```python
from build123d import *

# Parameters (mm, degrees)
EXTRUDE_3_DEPTH = 10
EXTRUDE_4_DEPTH = 20
SKETCH_6_W      = 120
SKETCH_6_H      = 120
EXTRUDE_5_DEPTH = 30


with BuildPart() as part:
    # 草圖1 → 填料-伸長3 (new body)
    with BuildSketch(Plane(origin=(0, 0, 0), x_dir=(1, 0, 0), z_dir=(0, 1, 0))):
        with BuildLine():
            Line((-60, 50), (60, 50))
            ThreePointArc((60, 50), (110, 0), (60, -50))
            Line((60, -50), (-60, -50))
            ThreePointArc((-60, -50), (-110, 0), (-60, 50))
        make_face()
        with BuildLine():
            Line((-60, -30), (60, -30))
            ThreePointArc((60, -30), (90, 0), (60, 30))
            Line((60, 30), (-60, 30))
            ThreePointArc((-60, 30), (-90, 0), (-60, -30))
        make_face(mode=Mode.SUBTRACT)
    extrude(amount=EXTRUDE_3_DEPTH)

    # 草圖4 → 填料-伸長4 (add)
    # profile 1 of 2: a face of its own
    with BuildSketch(Plane(origin=(0, 0, 0), x_dir=(1, 0, 0), z_dir=(0, 1, 0))):
        with BuildLine():
            Line((-60, 50), (60, 50))
            ThreePointArc((60, 50), (110, 0), (60, -50))
            Line((60, -50), (-60, -50))
            ThreePointArc((-60, -50), (-110, 0), (-60, 50))
        make_face()
        with BuildLine():
            ThreePointArc((60, -47), (107, 0), (60, 47))
            Line((60, 47), (-60, 47))
            ThreePointArc((-60, 47), (-107, 0), (-60, -47))
            Line((-60, -47), (60, -47))
        make_face(mode=Mode.SUBTRACT)
    # profile 2 of 2: a face of its own
    with BuildSketch(Plane(origin=(0, 0, 0), x_dir=(1, 0, 0), z_dir=(0, 1, 0))):
        with BuildLine():
            Line((-60, 33), (60, 33))
            ThreePointArc((60, 33), (93, 0), (60, -33))
            Line((60, -33), (-60, -33))
            ThreePointArc((-60, -33), (-93, 0), (-60, 33))
        make_face()
        with BuildLine():
            ThreePointArc((-60, 30), (-90, 0), (-60, -30))
            Line((-60, -30), (60, -30))
            ThreePointArc((60, -30), (90, 0), (60, 30))
            Line((60, 30), (-60, 30))
        make_face(mode=Mode.SUBTRACT)
    extrude(amount=EXTRUDE_4_DEPTH)

    # 草圖6 → 填料-伸長5 (add)
    with BuildSketch(Plane(origin=(0, 0, 0), x_dir=(1, 0, 0), z_dir=(0, 1, 0))):
        Rectangle(SKETCH_6_W, SKETCH_6_H)
    extrude(amount=-EXTRUDE_5_DEPTH)


solid = part.part
```
Verification items for the finished model (mm, model axes). A direction names the side the tool comes from. Coordinates: 2 decimals unless noted, no trailing zeros. Order: outer loops, then holes, each group sorted by start corner. A loop starts at its lowest first (then second) coordinate and runs counter-clockwise, first axis right, second up. Notation, with made-up numbers: (51.5, 24) -> (62.5, 24) arc R34 cw to (62.5, 61) -> close; hole circle Ø7 at (0.5, 27). An arc over 180 degrees is marked (long way). Put each result on its own line as item: value. Start each with the question number.
1) Cross-section at D-D (x = -49.5). Enter the section's corners in (y, z), plus the area to 3 significant figures.
2) Release check for a two-part mould opening along X. For faces 1 (the flat face through (-60, -15, 1)), 2 (the cylindrical face through (106.99, 14.93, 1.03)), 3 (the flat face through (-90.2, 0, -0.7)), 4 (the cylindrical face through (-89.993, 9.86, -0.66)) record: pulls with the +X half, pulls with the -X half, needs draft (parallel to the pull), parting line crosses it, or undercut.
3) Cross-section at A-A (z = 0). Enter the section's corners in (x, y), plus the area to 3 significant figures.
4) Go/stop test with flat-tipped pins: pin 1 (24 mm diameter, centred on y = -15.5, z = 13.5, fed in from +X); pin 2 (5 mm diameter, centred on x = -20, y = 16.5, fed in from -Z); pin 3 (22 mm diameter, centred on x = 7.5, y = 6.5, fed in from +Z); pin 4 (25 mm diameter, centred on x = -92.5, z = -13.5, fed in from -Y). Record where each tip stops, or that it passes through.
5) Cross-section at B-B (y = 2.5). Enter the section's corners in (x, z), plus the area to 3 significant figures.
6) Tool access check on faces 5 (the flat face through (-1, 10, -50)), 6 (the flat face through (-1, -15, -60)), 7 (the cylindrical face through (-92.99, 14.93, 0.73)), 8 (the flat face through (-1, -30, -1)), 9 (the flat face through (-1, 0, 55)). Record the directions out of +Z, -Z, +X, -X, +Y, -Y that give a thin tool (end or side, any length) a straight path to the whole face; none if there is none.
7) Cross-section at C-C (x = 64.5). Enter the section's corners in (y, z), plus the area to 3 significant figures.
8) Material ranges on L1, parallel to Z at x = -4.5, y = 0.5; L2, parallel to Z at x = 71.5, y = 13; L3, parallel to Z at x = -72, y = 13.5, recorded low to high.
Geometry check:
1. outline: (-30, -60) -> (0, -60) -> (0, -50) -> (20, -50) -> (20, -47) -> (10, -47) -> (10, -33) -> (20, -33) -> (20, -30) -> (0, -30) -> (0, 30) -> (20, 30) -> (20, 33) -> (10, 33) -> (10, 47) -> (20, 47) -> (20, 50) -> (0, 50) -> (0, 60) -> (-30, 60) -> close
1. area: 4,120 mm^2
2. face 1: pulls with the -X half
2. face 2: undercut
2. face 3: needs draft
2. face 4: undercut
3. outline: (-110, 0) -> (-90, 0) -> (-90, 20) -> (-93, 20) -> (-93, 10) -> (-107, 10) -> (-107, 20) -> (-110, 20) -> close; (-60, -30) -> (60, -30) -> (60, 0) -> (-60, 0) -> close; (90, 0) -> (110, 0) -> (110, 20) -> (107, 20) -> (107, 10) -> (93, 10) -> (93, 20) -> (90, 20) -> close
3. area: 4,120 mm^2
4. pin 1: stops at x = 60
4. pin 2: stops at z = -50
4. pin 3: stops at z = 60
4. pin 4: stops at y = 0
5. outline: (-60, -50) -> (60, -50) arc R50 ccw to (60, 50) -> (-60, 50) arc R50 ccw to start; hole (-60, -30) -> (60, -30) arc R30 ccw to (60, 30) -> (-60, 30) arc R30 ccw to start
5. area: 9,830 mm^2
6. face 5: -Z, +X, -X, +Y
6. face 6: -Z, +X, -X, +Y, -Y
6. face 7: +Y
6. face 8: +Z, -Z, +X, -X, -Y
6. face 9: +Z, +X, -X, +Y
7. outline: (0, -49.8) -> (20, -49.8) -> (20, -46.78) -> (10, -46.78) -> (10, -32.69) -> (20, -32.69) -> (20, -29.66) -> (0, -29.66) -> close; (0, 29.66) -> (20, 29.66) -> (20, 32.69) -> (10, 32.69) -> (10, 46.78) -> (20, 46.78) -> (20, 49.8) -> (0, 49.8) -> close
7. area: 524 mm^2
8. L1: z = -50 to -30, 30 to 50
8. L2: z = -48.66 to -45.57, -30.93 to -27.71, 27.71 to 30.93, 45.57 to 48.66
8. L3: z = -48.54 to -45.44, -30.74 to -27.5, 27.5 to 30.74, 45.44 to 48.54
